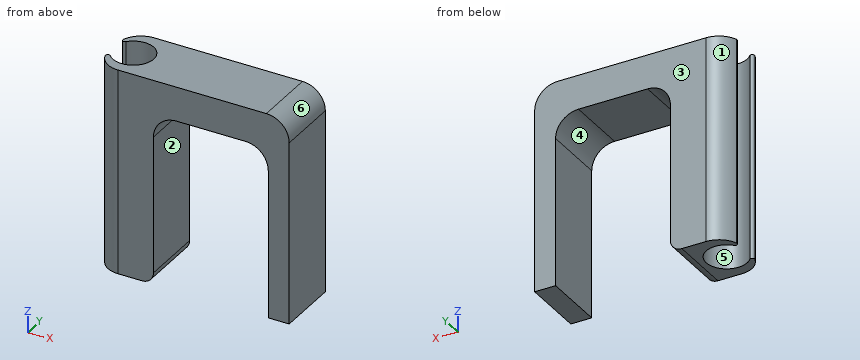
```python
from build123d import *

# Parameters (mm, degrees)
F1_DEPTH = 7
F2_R     = 4.55
F3_DEPTH = 45.721
F4_R     = 5.08
F5_R     = 0.5
F6_R     = 5.08
F7_R     = 2.54


with BuildPart() as f1:
    # F0 (on Front) → F1 (new body, symmetric)
    with BuildSketch(Plane.XZ):
        Polygon((21.59, 22.86), (-21.59, 22.86), (-21.59, -22.86), (-8.59, -22.86), (-8.59, 15.24), (16.937, 15.24), (16.937, -22.86), (21.59, -22.86), align=None)
    extrude(amount=F1_DEPTH, both=True)

    # F2 (on face) → F3 (cut, through all)
    with BuildSketch(Plane.XY.offset(22.86)):
        with Locations((-17.0908, 0)):
            Circle(F2_R)
    extrude(amount=-F3_DEPTH, mode=Mode.SUBTRACT)

    # F4
    f4_edges = [f1.edges().sort_by_distance(p)[0] for p in [
        (-8.59, 0, 15.24),
        (16.937, 0, 15.24),
        (-21.59, -7, 0),
        (-21.59, 7, 0),
    ]]
    fillet(f4_edges, radius=F4_R)

    # F5
    f5_edges = [f1.edges().sort_by_distance(p)[0] for p in [
        (-21.59, -0.678011, 0),
        (-21.59, 0.678011, 0),
    ]]
    fillet(f5_edges, radius=F5_R)

    # F6
    f6_edges = [f1.edges().sort_by_distance(p)[0] for p in [
        (21.59, 0, 22.86),
    ]]
    fillet(f6_edges, radius=F6_R)

    # F7
    f7_edges = [f1.edges().sort_by_distance(p)[0] for p in [
        (-8.59, 0, -22.86),
    ]]
    fillet(f7_edges, radius=F7_R)


solid = f1.part
```
Verification items for the finished model (mm, model axes). Face numbers are marked on the shaded views. A direction names the side the tool comes from. Coordinates: 2 decimals unless noted, no trailing zeros. Loops run counter-clockwise (first coordinate to the right, second up) from the corner with the lowest first, then second, coordinate; pieces in that order, holes last. Notation, with made-up numbers: (-40, 43.5) -> (-13, 43.5) arc R14 ccw to (-13, 61.5) -> close; hole circle Ø4 at (-39.75, -11.75). An arc over 180 degrees is marked (long way). Answer in a Markdown table with one row per item. Add a question column.
1. Section check A-A, the plane y = 0. Enter the section's corners in (x, z), then the cut area to 3 significant figures.
2. Draft check along X on the marked faces 3, 4, 5 and 6. Enter one of: +X half, -X half, draft (parallel to the pull), parting line (faces both ways), or undercut.
3. Material ranges on probe 1 along X at (y, z) = (0, 4.5); probe 2 along X at (y, z) = (3.5, -16); probe 3 along Z at (x, y) = (3, 2.75), recorded low to high. Write a range as [from, to].
4. Access from +Z, -Z, +X, -X, +Y, -Y to the whole of each face (thin tool, end or side, straight path). Record for the marked faces 1 and 2.
5. Section check B-B, the plane x = 8.5. Enter the section's corners in (y, z).
6. Depth check by flat-ended pin: P1, Ø6, axis at y = 1, z = -4, coming from the -X side; P2, Ø12, axis at x = -0.5, z = -5.5, coming from the +Y side; P3, Ø4, axis at x = 2, y = -2, coming from the -Z side. Enter the tip coordinate at first touch or a pass-through.
7. Section check C-C, the plane y = 6. Enter the section's corners in (x, z), then the cut area to 3 significant figures.
Derived:
| question | item | result |
|---|---|---|
| 1 | outline | (-12.54, -22.86) -> (-11.13, -22.86) arc R2.54 ccw to (-8.59, -20.32) -> (-8.59, 10.16) arc R5.08 cw to (-3.51, 15.24) -> (11.86, 15.24) arc R5.08 cw to (16.94, 10.16) -> (16.94, -22.86) -> (21.59, -22.86) -> (21.59, 17.78) arc R5.08 ccw to (16.51, 22.86) -> (-12.54, 22.86) -> close |
| 1 | area | 592 mm² |
| 2 | face 3 | draft |
| 2 | face 4 | undercut |
| 2 | face 5 | undercut |
| 2 | face 6 | +X half |
| 3 | probe 1 | x = [-12.54, -8.59], [16.94, 21.59] |
| 3 | probe 2 | x = [-21.34, -20], [-14.18, -8.59], [16.94, 21.59] |
| 3 | probe 3 | z = [15.24, 22.86] |
| 4 | face 1 | +Z, -Z, -X, +Y |
| 4 | face 2 | -Z, +Y, -Y |
| 5 | outline | (-7, 15.24) -> (7, 15.24) -> (7, 22.86) -> (-7, 22.86) -> close |
| 6 | P1 | stops at x = -21.36 |
| 6 | P2 | passes through |
| 6 | P3 | stops at z = 15.24 |
| 7 | outline | (-19.54, -22.86) -> (-11.13, -22.86) arc R2.54 ccw to (-8.59, -20.32) -> (-8.59, 10.16) arc R5.08 cw to (-3.51, 15.24) -> (11.86, 15.24) arc R5.08 cw to (16.94, 10.16) -> (16.94, -22.86) -> (21.59, -22.86) -> (21.59, 17.78) arc R5.08 ccw to (16.51, 22.86) -> (-19.54, 22.86) -> close |
| 7 | area | 912 mm² |
